The drawing under review shows one solid part. Ordinate dimensions are in mm from its lowest x, y, z. A direction names the side the tool comes from. Give positions to 0.01 mm unless a question says otherwise; leave off trailing zeros. Loops run counter-clockwise (first coordinate to the right, second up) from the corner with the lowest first, then second, coordinate; pieces in that order, holes last. Notation, with made-up numbers: (-8.5, 32) - (33.5, 32) arc R21 cw to (33.5, 62) - close; hole circle Ø5 at (-31.75, -16). An arc over 180 degrees is marked (long way). Put each result on its own line as item: value. Start each with the question number.
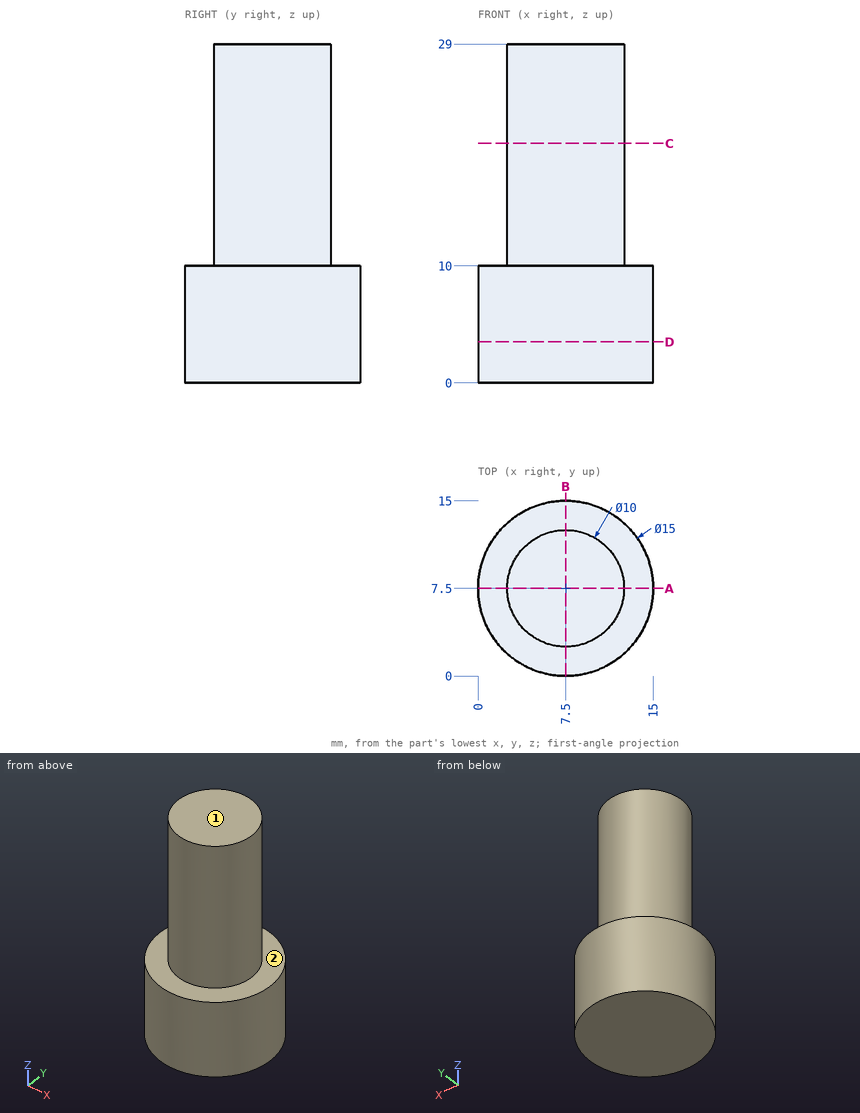
Item 1: Consider section C-C (z = 20.5). State the section outline as (x, y) points.
Item 2: Consider section D-D (z = 3.5). State the section outline as (x, y) points, plus the area to 3 significant figures.
Item 3: For L1, parallel to Y at x = 7.5, z = 18.25; L2, parallel to Z at x = 3.25, y = 12.75; L3, parallel to X at y = 2, z = 7, list the stretches that pass through material, from the lowest coordinate up. Write a range as from..to.
Item 4: Machinability: for the marked faces 1 and 2, which of the approach directions +Z, -Z, +X, -X, +Y, -Y give a long, thin tool a straight path to every point of the face, cutting with its end or side? Answer none if there is none.
Item 5: For P1, Ø1.5, axis at x = 8.5, z = 16, coming from the -Y side; P2, Ø4, axis at y = 10, z = 16, coming from the +X side; P3, Ø3, axis at y = 7, z = 25.5, coming from the -X side, all flat-tipped, find the tip position at first contact; note any pin that passes through.
Item 6: Consider section A-A (y = 7.5). State the section outline as (x, z) points.
Geometry says:
1. outline: circle Ø10 at (7.5, 7.5)
2. outline: circle Ø15 at (7.5, 7.5)
2. area: 177 mm2
3. L1: y = 2.5..12.5
3. L2: z = 0..10
3. L3: x = 2.4..12.6
4. face 1: +Z, +X, -X, +Y, -Y
4. face 2: +Z
5. P1: stops at y = 2.51
5. P2: stops at x = 12.47
5. P3: stops at x = 2.5
6. outline: (0, 0) - (15, 0) - (15, 10) - (12.5, 10) - (12.5, 29) - (2.5, 29) - (2.5, 10) - (0, 10) - close
